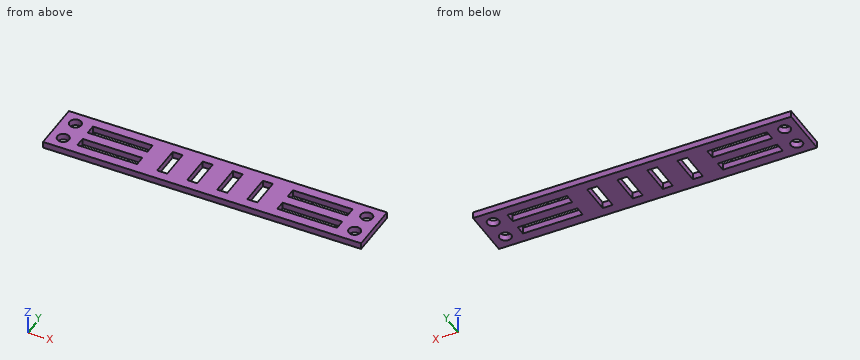
```python
from build123d import *

# Parameters (mm, degrees)
F0_W     = 95.25
F0_H     = 15
F0_R     = 1.75
F0_W_2   = 17.875
F0_H_2   = 3
F0_W_3   = 3
F0_H_3   = 9
F1_DEPTH = 1.92


with BuildPart() as f1:
    # F0 (on Top) → F1 (new body)
    with BuildSketch(Plane.XY):
        with Locations((47.625, 7.5)):
            Rectangle(F0_W, F0_H)
        with Locations((4, 4)):
            Circle(F0_R, mode=Mode.SUBTRACT)
        with Locations((17.6875, 4.5)):
            Rectangle(F0_W_2, F0_H_2, mode=Mode.SUBTRACT)
        with Locations((77.5625, 4.5)):
            Rectangle(F0_W_2, F0_H_2, mode=Mode.SUBTRACT)
        with Locations((91.25, 4)):
            Circle(F0_R, mode=Mode.SUBTRACT)
        with Locations((4, 11)):
            Circle(F0_R, mode=Mode.SUBTRACT)
        with Locations((17.6875, 10.5)):
            Rectangle(F0_W_2, F0_H_2, mode=Mode.SUBTRACT)
        with Locations((34.125, 7.5)):
            Rectangle(F0_W_3, F0_H_3, mode=Mode.SUBTRACT)
        with Locations((43.125, 7.5)):
            Rectangle(F0_W_3, F0_H_3, mode=Mode.SUBTRACT)
        with Locations((52.125, 7.5)):
            Rectangle(F0_W_3, F0_H_3, mode=Mode.SUBTRACT)
        with Locations((61.125, 7.5)):
            Rectangle(F0_W_3, F0_H_3, mode=Mode.SUBTRACT)
        with Locations((77.5625, 10.5)):
            Rectangle(F0_W_2, F0_H_2, mode=Mode.SUBTRACT)
        with Locations((91.25, 11)):
            Circle(F0_R, mode=Mode.SUBTRACT)
    extrude(amount=F1_DEPTH)


solid = f1.part
```
Design review of the part built by this model. Coordinates are the model's own, in mm. Round coordinates to 2 decimals unless told otherwise and drop trailing zeros. Write each loop counter-clockwise with the first axis right and the second up, starting at its lowest first coordinate (ties: lowest second). Pieces come first, ordered by that corner, then holes.
Item 1: We need section A-A on x = 61.5. Write out the cut boundary in (y, z).
Item 2: Clearance check with a flat-ended pin moving along its axis: pin 1 Ø1.5 at (x, y) = (19, 11) entering from -Z. State where the tip first meets the part, or that it passes through.
Item 3: For probe 1 along Y at (x, z) = (78.5, 1.3); probe 2 along Y at (x, z) = (4, 1.1); probe 3 along X at (y, z) = (8, 1.1) (3 decimals), list the stretches that pass through material, from the lowest coordinate up.
Item 4: We need section C-C on x = 77. Write out the cut boundary in (y, z).
Item 5: We need section B-B on y = 7.25. Write out the cut boundary in (x, z) (3 decimals), and give its area (3 significant figures).
Item 6: We need section D-D on x = 4. Write out the cut boundary in (y, z), and give its area (3 significant figures).
Returned:
1. outline: (0, 0) - (3, 0) - (3, 1.92) - (0, 1.92) - close; (12, 0) - (15, 0) - (15, 1.92) - (12, 1.92) - close
2. pin 1: passes through
3. probe 1: y = 0 to 3, 6 to 9, 12 to 15
3. probe 2: y = 0 to 2.25, 5.75 to 9.25, 12.75 to 15
3. probe 3: x = 0 to 32.625, 35.625 to 41.625, 44.625 to 50.625, 53.625 to 59.625, 62.625 to 95.25
4. outline: (0, 0) - (3, 0) - (3, 1.92) - (0, 1.92) - close; (6, 0) - (9, 0) - (9, 1.92) - (6, 1.92) - close; (12, 0) - (15, 0) - (15, 1.92) - (12, 1.92) - close
5. outline: (0, 0) - (32.625, 0) - (32.625, 1.92) - (0, 1.92) - close; (35.625, 0) - (41.625, 0) - (41.625, 1.92) - (35.625, 1.92) - close; (44.625, 0) - (50.625, 0) - (50.625, 1.92) - (44.625, 1.92) - close; (53.625, 0) - (59.625, 0) - (59.625, 1.92) - (53.625, 1.92) - close; (62.625, 0) - (95.25, 0) - (95.25, 1.92) - (62.625, 1.92) - close
5. area: 160 mm2
6. outline: (0, 0) - (2.25, 0) - (2.25, 1.92) - (0, 1.92) - close; (5.75, 0) - (9.25, 0) - (9.25, 1.92) - (5.75, 1.92) - close; (12.75, 0) - (15, 0) - (15, 1.92) - (12.75, 1.92) - close
6. area: 15.4 mm2
